Input: part model. Units: mm. Frame: model coordinates. Give positions to 0.01 mm unless a question says otherwise; leave off trailing zeros. Loops run counter-clockwise (first coordinate to the right, second up) from the corner with the lowest first, then second, coordinate; pieces in that order, holes last. Notation, with made-up numbers: (71, 24.5) - (111, 24.5) arc R10 ccw to (111, 36.5) - close; hole circle Ø2 at (40.5, 36.5). An arc over 180 degrees is marked (long way). Answer as a JSON object with one key per item and string values. Group by question number.
(1) Section query B-B (x = 54). Return loops of the section in (y, z), plus the area to 3 significant figures.
(2) Pin query (flat end, axial travel): P1, Ø12, axis at x = 92, y = 21, coming from the +Z side; P2, Ø8, axis at x = 84, z = -22.5, coming from the -Y side; P3, Ø8, axis at x = 86.5, y = 32, coming from the +Z side; P4, Ø12, axis at y = 35, z = -25.5, coming from the -X side. Return the tip coordinate at first contact, or that it passes through.
(3) Section query A-A (z = -12). Return loops of the section in (x, y), plus the area to 3 significant figures.
(4) Material intervals for L1, parallel to Z at x = 105, y = 36.5; L2, parallel to Z at x = 78.5, y = 31; L3, parallel to X at y = 17.5, z = -26.5, sorted ascending.
Solid Edge part; units mm, degrees
sketch "Sketch1" plane through (0, 0, 0) normal (0, -1, 0) x (1, 0, 0)
  line L0 (0, -37) -> (250, -37)
  line L1 (250, -37) -> (250, 0)
  line L2 (250, 0) -> (0, 0)
  line L3 (0, 0) -> (0, -37)
extrude "Protrusion1" add sketch "Sketch1" against normal blind 40
sketch "Sketch2" plane through (125, 0, -18.5) normal (0, -1, 0) x (1, 0, 0)
  arc A0 (10, 18.5) -> (-125, -2.2274) centre (10, -431.5) ccw
  line L0 (-125, -2.2274) -> (-125, 18.5)
  line L1 (-125, 18.5) -> (10, 18.5)
extrude "ExtrudedCutout_1" cut sketch "Sketch2" against normal blind 40
sketch "Sketch3" plane through (125, 0, -18.5) normal (0, -1, 0) x (1, 0, 0)
  line L0 (-125, -2.2274) -> (-33.462, 16.3963)
  line L1 (-33.462, 16.3963) -> (-125, 18.5)
  line L2 (-125, 18.5) -> (-125, -2.2274)
extrude "ExtrudedCutout_2" cut sketch "Sketch3" against normal blind 40
fillet "Round_1" radius 20 1 edges at (0, 20, -20.7274)
fillet "Round_2" radius 400 1 edges at (91.538, 20, -2.1037)
Recorded:
{
 "1": {"outline": "(0, -37) - (40, -37) - (40, -9.74) - (0, -9.74) - close", "area": "1,090 mm^2"},
 "2": {"P1": "stops at z = -2.44", "P2": "stops at y = 0", "P3": "stops at z = -3.35", "P4": "stops at x = 0.79"},
 "3": {"outline": "(42.9, 0) - (250, 0) - (250, 40) - (42.9, 40) - close", "area": "8,280 mm^2"},
 "4": {"L1": "z = -37 to -1.73", "L2": "z = -37 to -5.1", "L3": "x = 3.02 to 250"}
}
